from build123d import *

# Parameters (mm, degrees)
F1_R = 4


with BuildPart() as f2:
    # F2: sweep along a path in F0
    with BuildLine(Plane.XZ) as f2_path:
        Line((-260, 0), (-260, 42))
        ThreePointArc((-260, 42), (-258.242641, 46.242641), (-254, 48))
        Line((-254, 48), (254, 48))
        ThreePointArc((254, 48), (258.242641, 46.242641), (260, 42))
        Line((260, 42), (260, 0))
    # F1 (on Top) → F2 (sweep)
    with BuildSketch(Plane.XY):
        with Locations((-260, 0)):
            Circle(F1_R)
    sweep(path=f2_path.line)


solid = f2.part
The listing builds one solid part. Answer for the finished solid, in the listing's coordinates (mm). Give positions to 0.01 mm unless a question says otherwise; leave off trailing zeros. Use a Markdown table: item, result.
(1) Find the intervals of material crossed by probe 1 along X at (y, z) = (-0.5, 40.5); probe 2 along Z at (x, y) = (-196.5, 0.75); probe 3 along Z at (x, y) = (43, -0.25), in increasing order. Write a range as from..to.
Return value:
| item | result |
|---|---|
| probe 1 | -263.97..-256.03, 256.03..263.97 |
| probe 2 | 44.07..51.93 |
| probe 3 | 44.01..51.99 |
(2) Flat-ended cylindrical pins translate along their axes: P1, Ø3, axis at x = -23.5, y = -3, coming from the -Z side; P2, Ø1, axis at x = -121, y = -2, coming from the +Z side; P3, Ø4, axis at x = 121.5, y = 2.5, coming from the +Z side. Find the tip coordinate at first contact, or state that the pin passes through.
Return value:
| item | result |
|---|---|
| P1 | z = 44.29 |
| P2 | z = 51.71 |
| P3 | z = 51.97 |
(3) Determine the mould class of faces 1 (the cylindrical face through (-264, 0, 21)), 2 (the flat face through (-260, 0, 0)) for opening direction Y: released by +Y, released by -Y, zero draft, split by the parting line, or undercut.
Return value:
| item | result |
|---|---|
| face 1 | split by the parting line |
| face 2 | zero draft |
